Design review of the part built by this model. Coordinates are the model's own, in mm. Face numbers are marked on the shaded views. A direction names the side the tool comes from. Give positions to 0.01 mm unless a question says otherwise; leave off trailing zeros. Loops run counter-clockwise (first coordinate to the right, second up) from the corner with the lowest first, then second, coordinate; pieces in that order, holes last. Notation, with made-up numbers: (87, 23.25) - (143, 23.25) arc R21 ccw to (143, 28.25) - close; hole circle Ø4 at (8.25, -3.75). An arc over 180 degrees is marked (long way). Write each question's results on one line, items separated by ' | '.
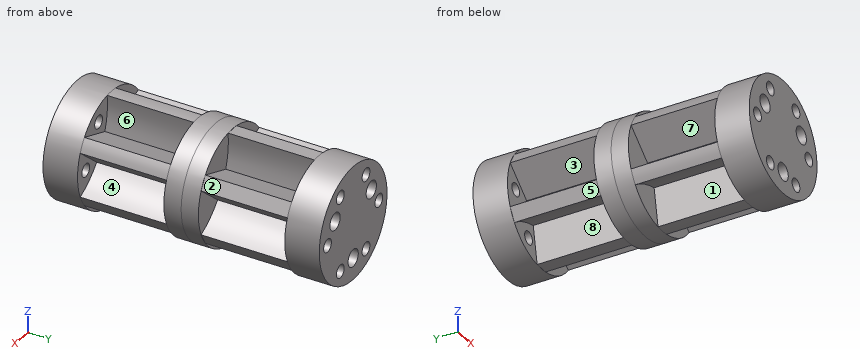
```python
from build123d import *
from build123d.topology import SkipClean

# Parameters (mm, degrees)
SKETCH_1_R               = 16.5
EXTRUDE_1_DEPTH          = 10
CUT_EXTRUDE_1_DEPTH      = 26.38700455
CUT_EXTRUDE_1_DEPTH_BACK = 26.38700455
SKETCH_4_R               = 2.5
SKETCH_4_R_2             = 1.9
EXTRUDE_2_DEPTH          = 25
SKETCH_7_R               = 16.5
EXTRUDE_3_DEPTH          = 5
EXTRUDE_4_DEPTH          = 25
SKETCH_10_R              = 16.5
EXTRUDE_5_DEPTH          = 10
SKETCH_11_R              = 1.9
SKETCH_11_R_2            = 2.5
CUT_EXTRUDE_3_DEPTH      = 10


with BuildPart() as part:
    # 草图1 → 凸台-拉伸1 (new body)
    with BuildSketch(Plane(origin=(0, 0, 0), x_dir=(1, 0, 0), z_dir=(0, 1, 0))):
        with Locations(Location((0, 0, 0), (0, 0, 270))):
            Circle(SKETCH_1_R)
    extrude(amount=EXTRUDE_1_DEPTH)

    # 草图4 → 切除-拉伸1 (cut, two sides: drawn at the far end of the back side and taken through both)
    with BuildSketch(Plane(origin=(0, 10, 0), x_dir=(1, 0, 0), z_dir=(0, 1, 0)).offset(-CUT_EXTRUDE_1_DEPTH_BACK)):
        with Locations(Location((0, 10.2, 0), (0, 0, 270))):
            Circle(SKETCH_4_R)
        with Locations(Location((-6.25, 10.825317547, 0), (0, 0, 270))):
            Circle(SKETCH_4_R_2)
        with Locations(Location((6.25, 10.825317547, 0), (0, 0, 270))):
            Circle(SKETCH_4_R_2)
        with Locations(Location((12.5, 0, 0), (0, 0, 270))):
            Circle(SKETCH_4_R_2)
        with Locations(Location((6.25, -10.825317547, 0), (0, 0, 270))):
            Circle(SKETCH_4_R_2)
        with Locations(Location((-6.25, -10.825317547, 0), (0, 0, 270))):
            Circle(SKETCH_4_R_2)
        with Locations(Location((-12.5, 0, 0), (0, 0, 270))):
            Circle(SKETCH_4_R_2)
        with Locations(Location((8.833459119, -5.1, 0), (0, 0, 270))):
            Circle(SKETCH_4_R)
        with Locations(Location((-8.833459119, -5.1, 0), (0, 0, 270))):
            Circle(SKETCH_4_R)
    extrude(amount=CUT_EXTRUDE_1_DEPTH + CUT_EXTRUDE_1_DEPTH_BACK, mode=Mode.SUBTRACT)

    # 草图6 → 凸台-拉伸2 (add)
    with SkipClean():  # the faces are left unmerged after this step: merging them gives an invalid solid
        with BuildSketch(Plane(origin=(0, 10, 0), x_dir=(1, 0, 0), z_dir=(0, 1, 0))):
            with BuildLine():
                Line((-15.206199095, -6.404803594), (-7.145587151, 0.449076957))
                ThreePointArc((-7.145587151, 0.449076957), (-10.83223207, 3.892058734), (-15.206199095, 6.404803594))
                ThreePointArc((-15.206199095, 6.404803594), (-14.289419162, 8.25), (-13.149822167, 9.966552914))
                ThreePointArc((-13.149822167, 9.966552914), (-8.786737771, 7.434958785), (-3.961705629, 5.96372152))
                Line((-3.961705629, 5.96372152), (-2.056376928, 16.371356508))
                ThreePointArc((-2.056376928, 16.371356508), (0, 16.5), (2.056376928, 16.371356508))
                Line((2.056376928, 16.371356508), (3.961705629, 5.96372152))
                ThreePointArc((3.961705629, 5.96372152), (8.786737771, 7.434958785), (13.149822167, 9.966552914))
                ThreePointArc((13.149822167, 9.966552914), (14.289419162, 8.25), (15.206199095, 6.404803594))
                ThreePointArc((15.206199095, 6.404803594), (10.83223207, 3.892058734), (7.145587151, 0.449076957))
                Line((7.145587151, 0.449076957), (15.206199095, -6.404803594))
                ThreePointArc((15.206199095, -6.404803594), (14.289419162, -8.25), (13.149822167, -9.966552914))
                Line((13.149822167, -9.966552914), (3.183881523, -6.412798476))
                ThreePointArc((3.183881523, -6.412798476), (2.045494299, -11.327017519), (2.056376928, -16.371356508))
                ThreePointArc((2.056376928, -16.371356508), (0, -16.5), (-2.056376928, -16.371356508))
                ThreePointArc((-2.056376928, -16.371356508), (-2.045494299, -11.327017519), (-3.183881523, -6.412798476))
                Line((-3.183881523, -6.412798476), (-13.149822167, -9.966552914))
                ThreePointArc((-13.149822167, -9.966552914), (-14.289419162, -8.25), (-15.206199095, -6.404803594))
            make_face()
        extrude(amount=EXTRUDE_2_DEPTH)

    # 草图7 → 凸台-拉伸3 (add)
    with SkipClean():  # the faces are left unmerged after this step: merging them gives an invalid solid
        with BuildSketch(Plane(origin=(0, 35, 0), x_dir=(1, 0, 0), z_dir=(0, 1, 0))):
            with Locations(Location((0, 0, 0), (0, 0, 270))):
                Circle(SKETCH_7_R)
        extrude_3 = extrude(amount=EXTRUDE_3_DEPTH)

    # 镜向3: 凸台-拉伸3 across plane
    with SkipClean():  # the faces are left unmerged after this step: merging them gives an invalid solid
        add(extrude_3.mirror(Plane.ZX.offset(40)))

    # 草图9 → 凸台-拉伸4 (add)
    with SkipClean():  # the faces are left unmerged after this step: merging them gives an invalid solid
        with BuildSketch(Plane(origin=(0, 45, 0), x_dir=(1, 0, 0), z_dir=(0, 1, 0))):
            with BuildLine():
                Line((-13.149822167, -9.966552914), (-3.183881523, -6.412798476))
                ThreePointArc((-3.183881523, -6.412798476), (-2.045494299, -11.327017519), (-2.056376928, -16.371356508))
                Line((-2.056376928, -16.371356508), (2.056376928, -16.371356508))
                ThreePointArc((2.056376928, -16.371356508), (2.045494299, -11.327017519), (3.183881523, -6.412798476))
                Line((3.183881523, -6.412798476), (13.149822167, -9.966552914))
                Line((13.149822167, -9.966552914), (15.206199095, -6.404803594))
                Line((15.206199095, -6.404803594), (7.145587151, 0.449076957))
                ThreePointArc((7.145587151, 0.449076957), (10.83223207, 3.892058734), (15.206199095, 6.404803594))
                Line((15.206199095, 6.404803594), (13.149822167, 9.966552914))
                ThreePointArc((13.149822167, 9.966552914), (8.786737771, 7.434958785), (3.961705629, 5.96372152))
                Line((3.961705629, 5.96372152), (2.056376928, 16.371356508))
                Line((2.056376928, 16.371356508), (-2.056376928, 16.371356508))
                Line((-2.056376928, 16.371356508), (-3.961705629, 5.96372152))
                ThreePointArc((-3.961705629, 5.96372152), (-8.786737771, 7.434958785), (-13.149822167, 9.966552914))
                Line((-13.149822167, 9.966552914), (-15.206199095, 6.404803594))
                ThreePointArc((-15.206199095, 6.404803594), (-10.83223207, 3.892058734), (-7.145587151, 0.449076957))
                Line((-7.145587151, 0.449076957), (-15.206199095, -6.404803594))
                Line((-15.206199095, -6.404803594), (-13.149822167, -9.966552914))
            make_face()
        extrude(amount=EXTRUDE_4_DEPTH)

    # 草图10 → 凸台-拉伸5 (add)
    with SkipClean():  # the faces are left unmerged after this step: merging them gives an invalid solid
        with BuildSketch(Plane(origin=(0, 70, 0), x_dir=(1, 0, 0), z_dir=(0, 1, 0))):
            with Locations(Location((0, 0, 0), (0, 0, 97.159326011))):
                Circle(SKETCH_10_R)
        extrude(amount=EXTRUDE_5_DEPTH)

    # 草图11 → 切除-拉伸3 (cut)
    with SkipClean():  # the faces are left unmerged after this step: merging them gives an invalid solid
        with BuildSketch(Plane(origin=(0, 80, 0), x_dir=(1, 0, 0), z_dir=(0, 1, 0))):
            with Locations(Location((12.5, 0, 0), (0, 0, 270))):
                Circle(SKETCH_11_R)
            with Locations(Location((8.833459119, -5.1, 0), (0, 0, 270))):
                Circle(SKETCH_11_R_2)
            with Locations(Location((6.25, -10.825317547, 0), (0, 0, 270))):
                Circle(SKETCH_11_R)
            with Locations(Location((-6.25, -10.825317547, 0), (0, 0, 270))):
                Circle(SKETCH_11_R)
            with Locations(Location((-8.833459119, -5.1, 0), (0, 0, 270))):
                Circle(SKETCH_11_R_2)
            with Locations(Location((-12.5, 0, 0), (0, 0, 270))):
                Circle(SKETCH_11_R)
            with Locations(Location((-6.25, 10.825317547, 0), (0, 0, 270))):
                Circle(SKETCH_11_R)
            with Locations(Location((0, 10.2, 0), (0, 0, 270))):
                Circle(SKETCH_11_R_2)
            with Locations(Location((6.25, 10.825317547, 0), (0, 0, 270))):
                Circle(SKETCH_11_R)
        extrude(amount=-CUT_EXTRUDE_3_DEPTH, mode=Mode.SUBTRACT)


solid = part.part
```
Item 1: We need section C-C on z = 11. Give the number of separate pieces and of enclosed holes in the cut face, then the cut area to 3 significant figures.
Output values:
separate pieces: 5 | enclosed holes: 0 | area: 795 mm²
Item 2: We need section B-B on y = 69. Give the boundary of the cut face in (x, z), then the cut area to 3 significant figures.
Output values:
outline: (-15.21, -6.4) - (-13.15, -9.97) arc R22 cw to (-3.96, -5.96) - (-2.06, -16.37) - (2.06, -16.37) - (3.96, -5.96) arc R22 cw to (13.15, -9.97) - (15.21, -6.4) arc R22 cw to (7.15, -0.45) - (15.21, 6.4) - (13.15, 9.97) - (3.18, 6.41) arc R22 cw to (2.06, 16.37) - (-2.06, 16.37) arc R22 cw to (-3.18, 6.41) - (-13.15, 9.97) - (-15.21, 6.4) - (-7.15, -0.45) arc R22 cw to start | area: 453 mm²
Item 3: Wall thickness on probe 1 along Y at (x, z) = (5, 13.5); probe 2 along X at (y, z) = (74, 0); probe 3 along X at (y, z) = (73.5, 6): over which ranges is each line inside the solid? List them lowest first.
Output values:
probe 1: y = 0 to 10, 35 to 45, 70 to 80 | probe 2: x = -16.5 to -14.4, -10.6 to 10.6, 14.4 to 16.5 | probe 3: x = -15.37 to -11.17, -6.5 to 6.5, 11.17 to 15.37
Item 4: Draft analysis for pull direction X (two halves, no side actions). For the marked faces 1, 2 and 3, state which applies: +X half, -X half, draft (parallel to the pull), parting line (faces both ways), or undercut.
Output values:
face 1: undercut | face 2: +X half | face 3: -X half
Item 5: Clearance check with flat-ended pins moving along their axes: P1, Ø8.5, axis at x = 7, z = -12, coming from the +Y side; P2, Ø3, axis at x = 6.25, z = -10.83, coming from the +Y side; P3, Ø1.5, axis at x = 8.5, z = 4.5, coming from the -Y side; P4, Ø1, axis at x = 1, y = 31.5, coming from the -Z side. State where each tip first meets the part, or that it passes through.
Output values:
P1: stops at y = 80 | P2: stops at y = 45 | P3: stops at y = 10 | P4: stops at z = -16.49
Item 6: Tool access review of the marked faces 4, 5, 6, 7 and 8: name each direction out of +Z, -Z, +X, -X, +Y, -Y from which nothing blocks a thin tool from reaching the whole face with its end or side.
Output values:
face 4: +X | face 5: -Z, -X | face 6: none | face 7: -X | face 8: -Z
Item 7: We need section A-A on y = 23. Give the boundary of the cut face in (x, z).
Output values:
outline: (-15.21, -6.4) arc R16.5 ccw to (-13.15, -9.97) arc R22 cw to (-3.96, -5.96) - (-2.06, -16.37) arc R16.5 ccw to (2.06, -16.37) - (3.96, -5.96) arc R22 cw to (13.15, -9.97) arc R16.5 ccw to (15.21, -6.4) arc R22 cw to (7.15, -0.45) - (15.21, 6.4) arc R16.5 ccw to (13.15, 9.97) - (3.18, 6.41) arc R22 cw to (2.06, 16.37) arc R16.5 ccw to (-2.06, 16.37) arc R22 cw to (-3.18, 6.41) - (-13.15, 9.97) arc R16.5 ccw to (-15.21, 6.4) - (-7.15, -0.45) arc R22 cw to start
